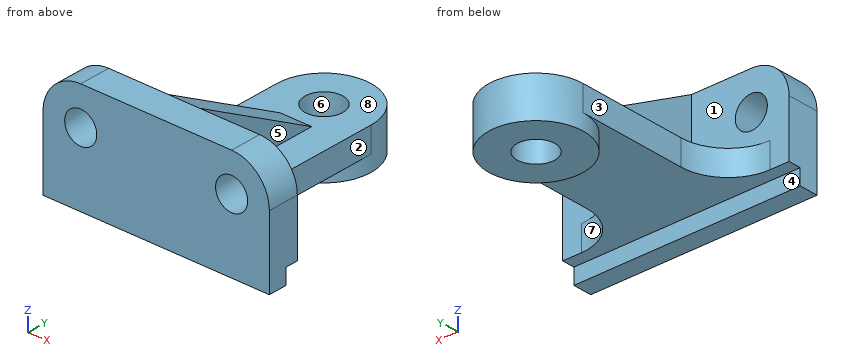
```python
from build123d import *

# Parameters (mm, degrees)
SKETCH1_W           = 72
SKETCH1_H           = 35
BOSS_EXTRUDE1_DEPTH = 10
FILLET1_R           = 12
SKETCH3_W           = 5
SKETCH3_H           = 4
CUT_EXTRUDE1_DEPTH  = 75.767974428
SKETCH4_R           = 6
BOSS_EXTRUDE2_DEPTH = 8
FILLET2_R           = 15
M12_TAPPED_HOLE1_D  = 10.2
SKETCH7_R           = 15
SKETCH7_R_2         = 6
BOSS_EXTRUDE3_DEPTH = 5
RIB1_REACH          = 87.013
SKETCH8_WALL_W      = 217.67731737
SKETCH8_WALL_H      = 10


with BuildPart() as part:
    # Sketch1 → Boss-Extrude1 (new body)
    with BuildSketch(Plane(origin=(0, 0, 0), x_dir=(1, 0, 0), z_dir=(0, 1, 0))):
        Rectangle(SKETCH1_W, SKETCH1_H)
    extrude(amount=BOSS_EXTRUDE1_DEPTH)

    # Fillet1
    fillet1_edges = [part.edges().sort_by_distance(p)[0] for p in [
        (36, 5, 17.5),
        (-36, 5, 17.5),
    ]]
    fillet(fillet1_edges, radius=FILLET1_R)

    # Sketch3 → Cut-Extrude1 (cut, through all)
    with BuildSketch(Plane(origin=(36, 0, 0), x_dir=(0, 0, -1), z_dir=(1, 0, 0))):
        with Locations((15, 8)):
            Rectangle(SKETCH3_W, SKETCH3_H)
    extrude(amount=-CUT_EXTRUDE1_DEPTH, mode=Mode.SUBTRACT)

    # Sketch4 → Boss-Extrude2 (add)
    with BuildSketch(Plane(origin=(0, 0, -12.5), x_dir=(-1, 0, 0), z_dir=(0, 0, -1))):
        with BuildLine():
            Line((-15, 10), (15, 10))
            Line((15, 10), (15, 60))
            ThreePointArc((15, 60), (0, 75), (-15, 60))
            Line((-15, 60), (-15, 10))
        make_face()
        with Locations((0, 60)):
            Circle(SKETCH4_R, mode=Mode.SUBTRACT)
    extrude(amount=-BOSS_EXTRUDE2_DEPTH)

    # Fillet2
    fillet2_edges = [part.edges().sort_by_distance(p)[0] for p in [
        (15, 10, -8.5),
        (-15, 10, -8.5),
    ]]
    fillet(fillet2_edges, radius=FILLET2_R)

    # M12 Tapped Hole1 (through all)
    with Locations(Plane(origin=(0, 10, 0), x_dir=(1, 0, 0), z_dir=(0, 1, 0))):
        with Locations((-24, -5.5), (24, -5.5)):
            Hole(M12_TAPPED_HOLE1_D / 2)

    # Sketch7 → Boss-Extrude3 (add)
    with BuildSketch(Plane(origin=(0, 0, -12.5), x_dir=(-1, 0, 0), z_dir=(0, 0, -1))):
        with Locations((0, 60)):
            Circle(SKETCH7_R)
        with Locations((0, 60)):
            Circle(SKETCH7_R_2, mode=Mode.SUBTRACT)
    extrude(amount=BOSS_EXTRUDE3_DEPTH)

    # Sketch8 wall → Rib1 (add, up to next)
    with BuildSketch(Plane(origin=(0, 30, 6.5), x_dir=(0, -0.876215908677, 0.481918749772), z_dir=(0, -0.481918749772, -0.876215908677)), mode=Mode.PRIVATE) as rib1_sk1:
        Rectangle(SKETCH8_WALL_W, SKETCH8_WALL_H)
    rib1_tool1 = extrude(rib1_sk1.sketch, amount=RIB1_REACH, mode=Mode.PRIVATE) - part.part
    add(rib1_tool1.solids().sort_by_distance((0, 30, 6.5))[0])


solid = part.part
```
Geometry: final body of the model. Coordinates: model frame, mm. Face numbers are marked on the shaded views. A direction names the side the tool comes from. Coordinates: 2 decimals unless noted, no trailing zeros. Order: outer loops, then holes, each group sorted by start corner. A loop starts at its lowest first (then second) coordinate and runs counter-clockwise, first axis right, second up.
Item 1: Draft query along X for the marked faces 6, 7 and 8. Return one class per face: released by +X, released by -X, zero draft, split by the parting line, or undercut.
Answer:
face 6: undercut
face 7: released by +X
face 8: zero draft
Item 2: Section query B-B (x = 0). Output: boundary loops of the cut face in (y, z), then the cut area to 3 significant figures.
Answer:
outline: (0, -17.5) - (6, -17.5) - (6, -12.5) - (45, -12.5) - (45, -17.5) - (54, -17.5) - (54, -4.5) - (50, -4.5) - (10, 17.5) - (0, 17.5) - close; (66, -17.5) - (75, -17.5) - (75, -4.5) - (66, -4.5) - close
area: 1,280 mm2
Item 3: Access query for the marked faces 1, 2, 3, 4 and 5. Directions: +Z, -Z, +X, -X, +Y, -Y. A direction counts if a zero-diameter tool reaches every point of the face in a straight line with its end or side. Return the directions, or none.
Answer:
face 1: +Z, -X, +Y
face 2: +Z, -Z, +X, +Y
face 3: +Z, -Z, -X, +Y
face 4: -Z, +X, -X
face 5: +Z, +X, +Y
Item 4: Contact query for flat-ended pins moving along their axis: P1, Ø2.5, axis at y = 51, z = -10, coming from the -X side; P2, Ø6.5, axis at y = 38.5, z = 7.5, coming from the -X side; P3, Ø16, axis at x = -1.5, y = 22, coming from the -Z side; P4, Ø17.5, axis at y = 24.5, z = 6, coming from the +X side. Output: stop coordinate, or through.
Answer:
P1: stops at x = -15
P2: passes through
P3: stops at z = -12.5
P4: stops at x = 5
Item 5: Section query C-C (y = 7). Output: boundary loops of the cut face in (x, z), then the cut area to 3 significant figures.
Answer:
outline: (-36, -12.5) - (36, -12.5) - (36, 5.5) arc R12 ccw to (24, 17.5) - (-24, 17.5) arc R12 ccw to (-36, 5.5) - close; hole circle Ø10.2 at (-24, 5.5); hole circle Ø10.2 at (24, 5.5)
area: 1,930 mm2
Item 6: Material intervals for line 1 along Y through (x, z) = (0, -13.25); line 2 along Z through (x, y) = (-24, 8); line 3 along Y through (x, z) = (-9, 7), sorted ascending.
Answer:
line 1: y = 0 to 6, 45 to 54, 66 to 75
line 2: z = -12.5 to 0.4, 10.6 to 17.5
line 3: y = 0 to 10
Item 7: Section query A-A (z = -14). Output: boundary loops of the cut face in (x, y), then the cut area to 3 significant figures.
Answer:
outline: (-36, 0) - (36, 0) - (36, 6) - (-36, 6) - close; circle Ø30 at (0, 60); hole circle Ø12 at (0, 60)
area: 1,030 mm2
Item 8: Section query D-D (z = -9). Output: boundary loops of the cut face in (x, y), then the cut area to 3 significant figures.
Answer:
outline: (-36, 0) - (36, 0) - (36, 10) - (30, 10) arc R15 cw to (15, 25) - (15, 60) arc R15 ccw to (-15, 60) - (-15, 25) arc R15 cw to (-30, 10) - (-36, 10) - close; hole circle Ø12 at (0, 60)
area: 2,560 mm2
